```python
from build123d import *

# Parameters (mm, degrees)
SKETCH_1_R               = 1.6
EXTRUDE_1_DEPTH          = 1
FILLET_2_R               = 4
CUT_EXTRUDE_1_DEPTH      = 51.042481953
CUT_EXTRUDE_1_DEPTH_BACK = 51.042481953


with BuildPart() as part:
    # 草图1 → 凸台-拉伸1 (new, symmetric)
    with BuildSketch(Plane(origin=(0, 0, 0), x_dir=(1, 0, 0), z_dir=(0, 1, 0))):
        with BuildLine():
            ThreePointArc((-24, -32), (0, -8), (24, -32))
            Line((24, -32), (32.5, -32))
            Line((32.5, -32), (32.5, 32))
            Line((32.5, 32), (24, 32))
            Line((24, 32), (24, 38))
            Line((24, 38), (-24, 38))
            Line((-24, 38), (-24, 32))
            Line((-24, 32), (-32.5, 32))
            Line((-32.5, 32), (-32.5, -32))
            Line((-32.5, -32), (-24, -32))
        make_face()
        with Locations(Location((-20.506096654, -11.493903346, 0), (0, 0, 270))):
            Circle(SKETCH_1_R, mode=Mode.SUBTRACT)
        with Locations(Location((20.506096654, -11.493903346, 0), (0, 0, 270))):
            Circle(SKETCH_1_R, mode=Mode.SUBTRACT)
        with Locations(Location((-6, 20, 0), (0, 0, 270))):
            Circle(SKETCH_1_R, mode=Mode.SUBTRACT)
        with Locations(Location((-16, 28, 0), (0, 0, 270))):
            Circle(SKETCH_1_R, mode=Mode.SUBTRACT)
        with Locations(Location((0, -3, 0), (0, 0, 270))):
            Circle(SKETCH_1_R, mode=Mode.SUBTRACT)
        with Locations(Location((6, 20, 0), (0, 0, 270))):
            Circle(SKETCH_1_R, mode=Mode.SUBTRACT)
        with Locations(Location((16, 28, 0), (0, 0, 270))):
            Circle(SKETCH_1_R, mode=Mode.SUBTRACT)
        with Locations(Location((18, 35, 0), (0, 0, 270))):
            Circle(SKETCH_1_R, mode=Mode.SUBTRACT)
        with Locations(Location((-18, 35, 0), (0, 0, 270))):
            Circle(SKETCH_1_R, mode=Mode.SUBTRACT)
    extrude(amount=EXTRUDE_1_DEPTH, both=True)

    # 圆角2
    fillet_2_edges = [part.edges().sort_by_distance(p)[0] for p in [
        (32.5, 0, 32),
        (24, 0, 32),
        (-24, 0, 32),
        (-32.5, 0, 32),
    ]]
    fillet(fillet_2_edges, radius=FILLET_2_R)

    # 草图2 → 切除-拉伸1 (cut, two sides: drawn at the far end of the back side and taken through both)
    with BuildSketch(Plane(origin=(0, 1, 0), x_dir=(1, 0, 0), z_dir=(0, 1, 0)).offset(-CUT_EXTRUDE_1_DEPTH_BACK)):
        Polygon((32.5, 32), (24, 32), (32.5, -4), align=None)
        Polygon((-32.5, -4), (-32.5, 32), (-24, 32), align=None)
    extrude(amount=CUT_EXTRUDE_1_DEPTH + CUT_EXTRUDE_1_DEPTH_BACK, mode=Mode.SUBTRACT)


solid = part.part
```
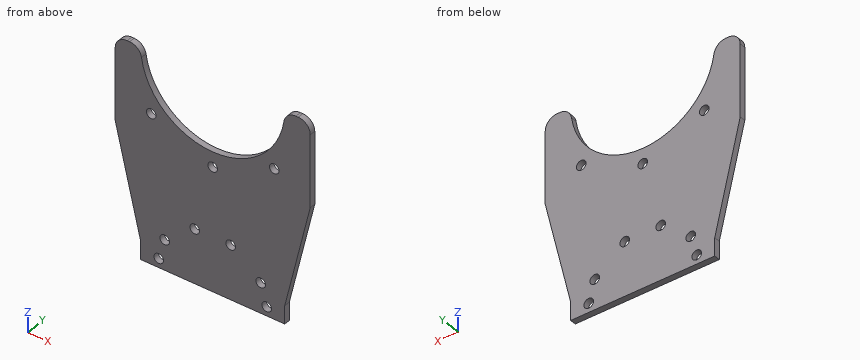
Input: part model. Units: mm. Frame: model coordinates. Round coordinates to 2 decimals unless told otherwise and drop trailing zeros. Order: outer loops, then holes, each group sorted by start corner. A loop starts at its lowest first (then second) coordinate and runs counter-clockwise, first axis right, second up. Notation, with made-up numbers: (-25, -11.5) - (-13, -11.5) arc R28 cw to (-13, 8.5) - close; hole circle Ø6 at (62, 20.25). An arc over 180 degrees is marked (long way). One line per question, with ' | ' between items. Start each with the question number.
1) Ray query, probe 1 along X at (y, z) = (0.7, -28); probe 2 along X at (y, z) = (-0.4, -34); probe 3 along X at (y, z) = (0.15, 19.5). Return the intervals inside material, ascending.
2) Cut plane C-C, the plane z = 14. Return the cut outline in (x, y), then the cut area to 3 significant figures.
3) Cut plane D-D, the plane y = 0.1. Give the number of separate pieces and of enclosed holes in the cut face, then the cut area to 3 significant figures.
4) Cut plane A-A, the plane x = 0. Return the cut outline in (y, z), then the cut area to 3 significant figures.
5) Contact query for flat-ended pins moving along their axis: P1, Ø1, axis at x = -19.5, y = 0, coming from the +Z side; P2, Ø1, axis at y = 0, z = -36.5, coming from the +X side. Output: stop coordinate, or through.
6) Cut plane B-B, the plane z = -35. Return the cut outline in (x, y).
Worked out:
1) probe 1: x = -24.94 to -17.6, -14.4 to 14.4, 17.6 to 24.94 | probe 2: x = -24 to -19.25, -16.75 to 16.75, 19.25 to 24 | probe 3: x = -32.5 to -20.49, 20.49 to 32.5
2) outline: (-32.5, -1) - (-15.87, -1) - (-15.87, 1) - (-32.5, 1) - close; (15.87, -1) - (32.5, -1) - (32.5, 1) - (15.87, 1) - close | area: 66.5 mm^2
3) separate pieces: 1 | enclosed holes: 9 | area: 3,150 mm^2
4) outline: (-1, -38) - (1, -38) - (1, 1.4) - (-1, 1.4) - close; (-1, 4.6) - (1, 4.6) - (1, 8) - (-1, 8) - close | area: 85.6 mm^2
5) P1: stops at z = 18.73 | P2: stops at x = 24
6) outline: (-24, -1) - (-19.6, -1) - (-19.6, 1) - (-24, 1) - close; (-16.4, -1) - (16.4, -1) - (16.4, 1) - (-16.4, 1) - close; (19.6, -1) - (24, -1) - (24, 1) - (19.6, 1) - close
